Part model, mm, in its own coordinate system. A direction names the side the tool comes from. Coordinates: 2 decimals unless noted, no trailing zeros. Write each loop counter-clockwise with the first axis right and the second up, starting at its lowest first coordinate (ties: lowest second). Pieces come first, ordered by that corner, then holes. Notation, with made-up numbers: M -15,-36.5 L -7,-36.5 A27 cw -7,-12.5 Z; hole C -21.5,-1 d7. An arc over 180 degrees is marked long. Use a Markdown table: item, result. Add a question column.
Q1. Tool access for faces 4 (the flat face through (0.5, 45.4, 12.6)), 5 (the cylindrical face through (-107.797, 58.859, 12.325)), 6 (the flat face through (-45.82, 59.49, 10.99)), 7 (the cylindrical face through (-0.9, 58.14, 12.32)): list every direction of +Z, -Z, +X, -X, +Y, -Y with a clear straight run to the whole face (end or side of a thin tool).
Q2. Wall check: L1, parallel to Z at x = 0.8, y = 5; L2, parallel to X at y = 44, z = 3.5; L3, parallel to Y at x = 0.6, z = 19. Give the ranges that are in metal, low to high. Write a range as from..to.
Q3. Pin check, flat tips, straight feed: pin 1 Ø1.1 at (x, z) = (-108.5, 16.5) entering from +Y; pin 2 Ø1 at (x, z) = (-71.5, 22) entering from -Y; pin 3 Ø1.1 at (y, z) = (59.5, 12.5) entering from +X. Stop position of each tip, or through.
Q4. Slice it at C-C on y = 41.5. Write the cut outline in (x, z).
Q5. Slice it at A-A on y = 24. Write the cut outline in (x, z).
Q6. Slice it at B-B on x = -74.5. Write the cut outline in (y, z).
Q7. Slice it at D-D on z = 11. Count the separate pieces of the cut face and the enclosed holes in it, then the cut area to 3 significant figures.
Q8. Mould opens along Y. For faces 1 (the flat face through (-59.99, 59.49, 11.18)), 2 (the flat face through (-108.5, 15.1, 8.9)), 3 (the flat face through (-55, 59, 18)) say: released by +Y, released by -Y, zero draft, split by the parting line, or undercut.
from build123d import *

# Parameters (mm, degrees)
F1_DEPTH = 25
F3_DEPTH = 25
F5_DEPTH = 200


with BuildPart() as f1:
    # F0 (on Top) → F1 (new body)
    with BuildSketch(Plane.XY):
        with BuildLine():
            Line((0, 56), (0, 0))
            Line((0, 0), (1, 0))
            Line((1, 0), (1, 56))
            ThreePointArc((1, 56), (-0.1715728753, 58.8284271247), (-3, 60))
            Line((-3, 60), (-105, 60))
            ThreePointArc((-105, 60), (-107.8284271247, 58.8284271247), (-109, 56))
            Line((-109, 56), (-109, 0))
            Line((-109, 0), (-108, 0))
            Line((-108, 0), (-108, 56))
            ThreePointArc((-108, 56), (-107.1213203436, 58.1213203436), (-105, 59))
            Line((-105, 59), (-3, 59))
            ThreePointArc((-3, 59), (-0.8786796564, 58.1213203436), (0, 56))
        make_face()
    extrude(amount=F1_DEPTH)

    # F2 (on face) → F3 (cut)
    with BuildSketch(Plane.XZ.offset(-59)):
        Polygon((-55.8284271247, 21), (-84.1715728753, 21), (-70, 6.8284271247), align=None)
        Polygon((-36, 6.8284271247), (-21.8284271247, 21), (-50.1715728753, 21), align=None)
        Polygon((-101.1715728753, 4), (-72.8284271247, 4), (-87, 18.1715728753), align=None)
        Polygon((-104, 21), (-104, 6.8284271247), (-89.8284271247, 21), align=None)
        Polygon((-67.1715728753, 4), (-38.8284271247, 4), (-53, 18.1715728753), align=None)
        Polygon((-10.4142135624, 9.5857864376), (-19, 18.1715728753), (-33.1715728753, 4), (-4.8284271247, 4), align=None)
    extrude(amount=-F3_DEPTH, mode=Mode.SUBTRACT)

    # F4 (on face) → F5 (cut)
    with BuildSketch(Plane(origin=(-109, 0, 0), x_dir=(0, -1, 0), z_dir=(-1, 0, 0))):
        with BuildLine():
            ThreePointArc((-5, 21), (-6.4142135624, 17.5857864376), (-3, 19))
            ThreePointArc((-3, 19), (-3.5857864376, 20.4142135624), (-5, 21))
        make_face()
        with BuildLine():
            ThreePointArc((-3, 6), (-6.4142135624, 7.4142135624), (-5, 4))
            ThreePointArc((-5, 4), (-3.5857864376, 4.5857864376), (-3, 6))
        make_face()
        Polygon((-10, 14), (-10, 21), (-37, 21), (-20, 4), align=None)
        Polygon((-20, 4), (-37, 21), (-54, 4), align=None)
    extrude(amount=-F5_DEPTH, mode=Mode.SUBTRACT)


solid = f1.part
Recorded:
| question | item | result |
|---|---|---|
| 1 | face 4 | +X, -X |
| 1 | face 5 | +Z, -Z, -X, +Y |
| 1 | face 6 | +Y, -Y |
| 1 | face 7 | +Z, -Z, -Y |
| 2 | L1 | 0..4, 8..17, 21..25 |
| 2 | L2 | -109..-108, 0..1 |
| 2 | L3 | 0..3, 7..10, 39..57.74 |
| 3 | pin 1 | y = 58.7 |
| 3 | pin 2 | y = 59 |
| 3 | pin 3 | x = -0.3 |
| 4 | outline | M -109,0 L -108,0 L -108,4 L -109,4 Z; M -109,16.5 L -108,16.5 L -108,25 L -109,25 Z; M 0,0 L 1,0 L 1,4 L 0,4 Z; M 0,16.5 L 1,16.5 L 1,25 L 0,25 Z |
| 5 | outline | M -109,0 L -108,0 L -108,4 L -109,4 Z; M -109,21 L -108,21 L -108,25 L -109,25 Z; M 0,0 L 1,0 L 1,4 L 0,4 Z; M 0,21 L 1,21 L 1,25 L 0,25 Z |
| 6 | outline | M 59,0 L 60,0 L 60,4 L 59,4 Z; M 59,5.67 L 60,5.67 L 60,11.33 L 59,11.33 Z; M 59,21 L 60,21 L 60,25 L 59,25 Z |
| 7 | separate pieces | 9 |
| 7 | enclosed holes | 0 |
| 7 | area | 93.1 mm² |
| 8 | face 1 | zero draft |
| 8 | face 2 | undercut |
| 8 | face 3 | released by -Y |
